Here's the drawing with two shaded views (mm, measured from the low corner). I have some questions. A direction names the side the tool comes from. Coordinates: 2 decimals unless noted, no trailing zeros. Write each loop counter-clockwise with the first axis right and the second up, starting at its lowest first coordinate (ties: lowest second). Pieces come first, ordered by that corner, then holes. Notation, with made-up numbers: (-37.75, -2.5) -> (21.25, -2.5) arc R20 cw to (21.25, 23.5) -> close; hole circle Ø3 at (47, -12). An arc over 180 degrees is marked (long way). Use one line per item in the form item = value.
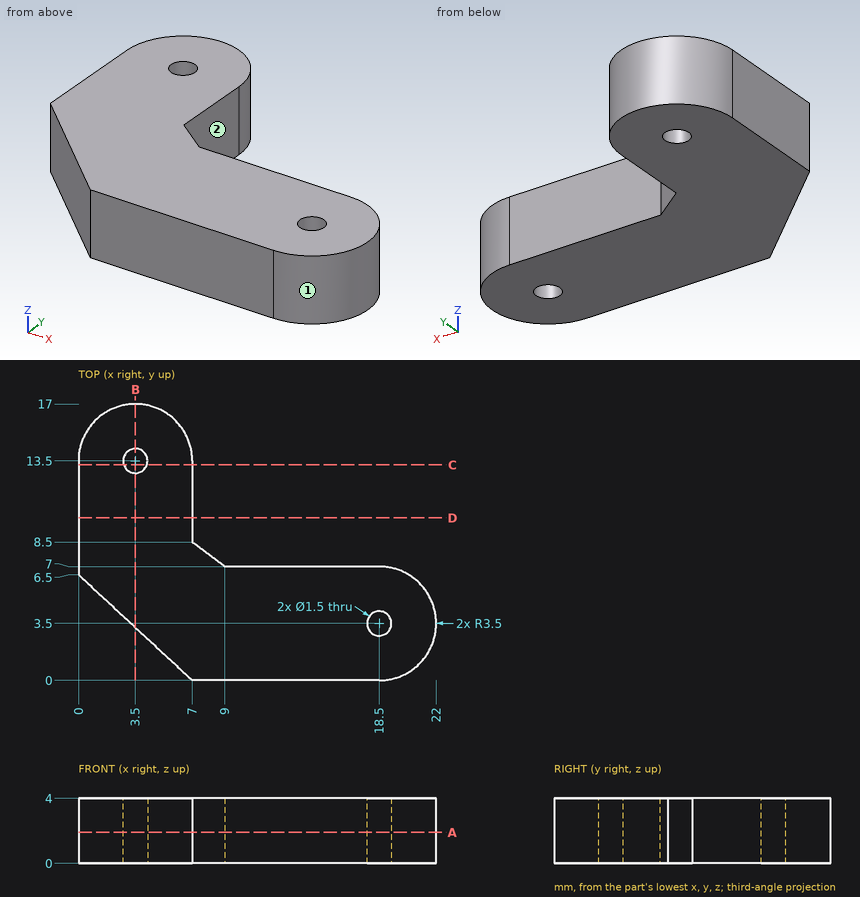
Q1. Will this pin go through, and if not, where does the flat tip stop? pin 1 (2 mm diameter, centred on x = 13.5, z = 3, fed in from +Y).
Return value:
pin_1 = 7
Q2. Suppose I cut it at D-D (y = 10). Write out the boundary of the cut face in (x, z), then the cut area to 3 significant figures.
Return value:
outline = (0, 0) -> (7, 0) -> (7, 4) -> (0, 4) -> close
area = 28.0 mm2
Q3. Suppose I cut it at C-C (y = 13.25). Write out the boundary of the cut face in (x, z).
Return value:
outline = (0, 0) -> (2.79, 0) -> (2.79, 4) -> (0, 4) -> close; (4.21, 0) -> (7, 0) -> (7, 4) -> (4.21, 4) -> close
Q4. Suppose I cut it at A-A (z = 1.9). Write out the boundary of the cut face in (x, y).
Return value:
outline = (0, 6.5) -> (7, 0) -> (18.5, 0) arc R3.5 ccw to (18.5, 7) -> (9, 7) -> (7, 8.5) -> (7, 13.5) arc R3.5 ccw to (0, 13.5) -> close; hole circle Ø1.5 at (3.5, 13.5); hole circle Ø1.5 at (18.5, 3.5)
Q5. If I drill on line 1 (Y direction, x = 18.5, z = 1.3); line 2 (X direction, y = 12.25, z = 2.05), over which ranges is the centre line in solid material (lowest first)? Write a range as from..to.
Return value:
line_1 = 0..2.75, 4.25..7
line_2 = 0..7
Q6. Suppose I cut it at B-B (x = 3.5). Write out the boundary of the cut face in (y, z), then the cut area to 3 significant figures.
Return value:
outline = (3.25, 0) -> (12.75, 0) -> (12.75, 4) -> (3.25, 4) -> close; (14.25, 0) -> (17, 0) -> (17, 4) -> (14.25, 4) -> close
area = 49.0 mm2
Q7. For the marked faces 1 and 2, which set-ups out of +Z, -Z, +X, -X, +Y, -Y let a thin tool reach every point of the face, with its end or its side?
Return value:
face_1 = +Z, -Z, +X
face_2 = +Z, -Z, +X, +Y
